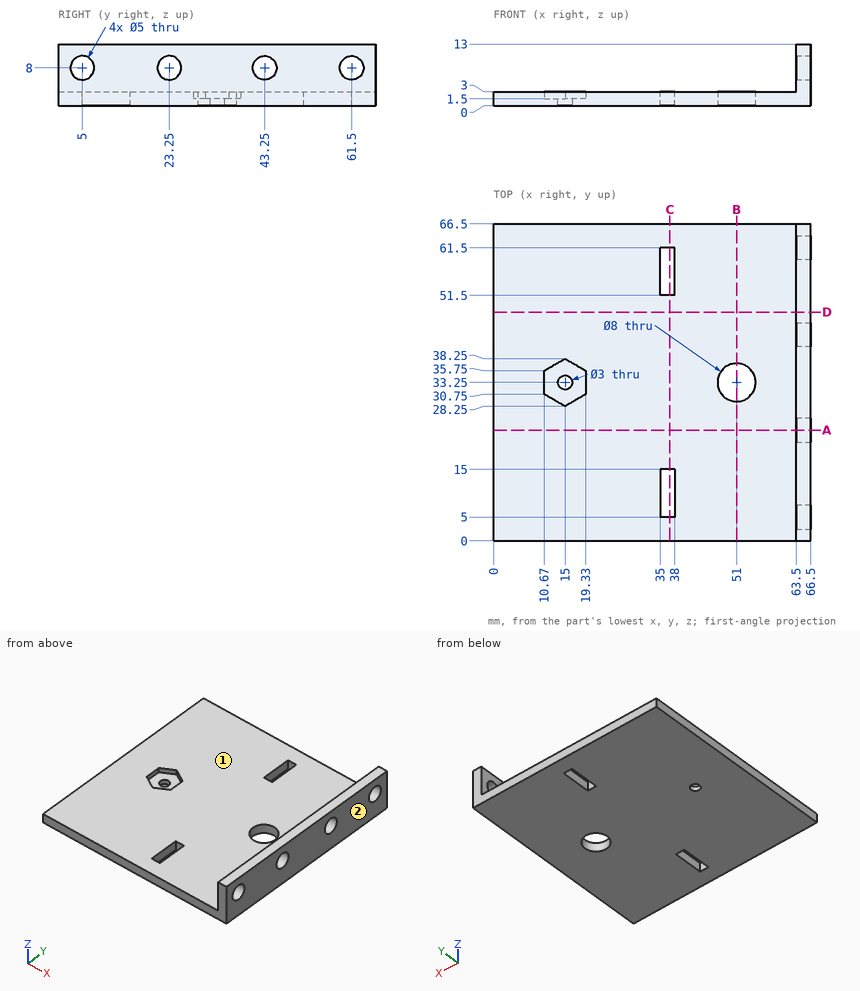
For this review, use the dimensioned drawing (mm, ordinates from the lowest corner) and the shaded views. A direction names the side the tool comes from. Give positions to 0.01 mm unless a question says otherwise; leave off trailing zeros. Order: outer loops, then holes, each group sorted by start corner. A loop starts at its lowest first (then second) coordinate and runs counter-clockwise, first axis right, second up. Notation, with made-up numbers: (32, -38.75) - (68, -38.75) arc R21 ccw to (68, -8.75) - close; hole circle Ø2 at (7.5, 64). An arc over 180 degrees is marked (long way). Use CSV: the item, a comma, the result in double quotes. Start each with the question number.
Q1. We need section B-B, the plane x = 51. Write out the cut boundary in (y, z), and give its area (4 significant figures).
Q2. We need section D-D, the plane y = 48. Write out the cut boundary in (x, z), and give its area (4 significant figures).
Q3. To check wall thickness, follow line 1 along Z through (x, y) = (65.6, 5); line 2 along Y through (x, z) = (15, 0.3); line 3 along X through (y, z) = (46, 12.25). State the ranges of each line that lie inside material, in increasing order. Write a range as [from, to].
Q4. We need section C-C, the plane x = 37. Write out the cut boundary in (y, z).
Q5. Tool access review of the marked faces 1 and 2: name each direction out of +Z, -Z, +X, -X, +Y, -Y from which nothing blocks a thin tool from reaching the whole face with its end or side.
Q6. Clearance check with flat-ended pins moving along their axes: pin 1 Ø6.5 at (y, z) = (5, 8) entering from +X; pin 2 Ø6.5 at (y, z) = (61.5, 8) entering from -X; pin 3 Ø7 at (x, y) = (16, 34) entering from +Z. State where each tip first meets the part, or that it passes through.
Q7. We need section A-A, the plane y = 23.25. Write out the cut boundary in (x, z), and give its area (4 significant figures).
Outcome:
1,outline,"(0, 0) - (29.25, 0) - (29.25, 3) - (0, 3) - close; (37.25, 0) - (66.5, 0) - (66.5, 3) - (37.25, 3) - close"
1,area,"175.5 mm^2"
2,outline,"(0, 0) - (66.5, 0) - (66.5, 13) - (63.5, 13) - (63.5, 3) - (0, 3) - close"
2,area,"229.5 mm^2"
3,line 1,"z = [0, 5.5], [10.5, 13]"
3,line 2,"y = [0, 31.75], [34.75, 66.5]"
3,line 3,"x = [63.5, 66.5]"
4,outline,"(0, 0) - (5, 0) - (5, 3) - (0, 3) - close; (15, 0) - (51.5, 0) - (51.5, 3) - (15, 3) - close; (61.5, 0) - (66.5, 0) - (66.5, 3) - (61.5, 3) - close"
5,face 1,"+Z, -X, +Y, -Y"
5,face 2,"+Z, -Z, +X, +Y, -Y"
6,pin 1,"stops at x = 66.5"
6,pin 2,"stops at x = 63.5"
6,pin 3,"stops at z = 3"
7,outline,"(0, 0) - (66.5, 0) - (66.5, 5.5) - (63.5, 5.5) - (63.5, 3) - (0, 3) - close; (63.5, 10.5) - (66.5, 10.5) - (66.5, 13) - (63.5, 13) - close"
7,area,"214.5 mm^2"
